The listing builds one solid part. Answer for the finished solid, in the listing's coordinates (mm). Face numbers are marked on the shaded views. Give positions to 0.01 mm unless a question says otherwise; leave off trailing zeros. Loops run counter-clockwise (first coordinate to the right, second up) from the corner with the lowest first, then second, coordinate; pieces in that order, holes last. Notation, with made-up numbers: M 67,74.25 L 81,74.25 A20 ccw 81,86.25 Z; hole C 39.5,-2.5 d4. An arc over 180 degrees is marked long. Return JSON: item names as keys, results as strings.
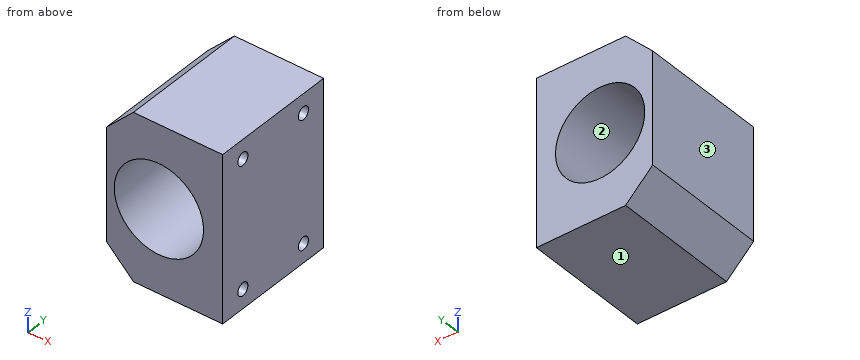
Autodesk Inventor part; units mm, degrees
ref_plane "YZ Plane" through (0, 0, 0) normal (1, 0, 0) x (0, 1, 0)
ref_plane "XZ Plane" through (0, 0, 0) normal (0, 1, 0) x (-1, 0, 0)
ref_plane "XY Plane" through (0, 0, 0) normal (0, 0, 1) x (1, 0, 0)
sketch "Sketch1" plane through (0, 0, 0) normal (0, 1, 0) x (-1, 0, 0)
  circle A0 centre (0, 0) radius 14
  line L0 (0, 0) -> (-20, 0)
  line L1 (-20, 0) -> (-20, -26)
  line L2 (-20, -26) -> (8, -26)
  line L3 (8, -26) -> (16.4853, -17.5147)
  line L4 (-20, 0) -> (-20, 26)
  line L5 (-20, 26) -> (8, 26)
  line L6 (8, 26) -> (16.4853, 17.5147)
  line L7 (16.4853, 17.5147) -> (16.4853, -17.5147)
  dimension "d0" = 28
  dimension "d1" = 20
  dimension "d2" = 26
  dimension "d3" = 28
  dimension "d4" = 12
  dimension "d5" = 135
  dimension "d6" = 28
  dimension "d7" = 26
  dimension "d8" = 12
extrude "Extrusion1" add sketch "Sketch1" along normal blind 40
sketch "Sketch2" plane through (20, 0, 26) normal (1, 0, 0) x (0, 0, -1)
  line L0 (0, 0) -> (0, 40)
  line L1 (0, 40) -> (0, 32)
  circle A0 centre (6, 32) radius 2
  point P0 (26, 0)
  dimension "d11" = 8
  dimension "d13" = 4
extrude "Extrusion2" cut sketch "Sketch2" against normal blind 15
pattern_linear "Rectangular Pattern1" count 2 spacing 24 along (0, -1, 0) count 2 spacing 40 along (0, 0, -1) of "Extrusion2"
properties part number "Soporte Tuerca"
(1) Straight lines are drawn through the part: line 1 along Y through (x, z) = (8.25, 20); line 2 along Y through (x, z) = (7.5, 21.5); line 3 along Z through (x, y) = (0, 11). For each, find the intervals that lie inside material, in ascending order.
Values follow:
{"line 1": "0 to 6, 10 to 30, 34 to 40", "line 2": "0 to 6.68, 9.32 to 30.68, 33.32 to 40", "line 3": "-26 to -14, 14 to 26"}
(2) The part is cut by section A-A (x = 0). Determine the outline of the cut face in (y, z), and give its area (3 significant figures).
Values follow:
{"outline": "M 0,-26 L 40,-26 L 40,-14 L 0,-14 Z; M 0,14 L 40,14 L 40,26 L 0,26 Z", "area": "960 mm²"}
(3) The part is cut by section C-C (z = 0). Determine the outline of the cut face in (x, y).
Values follow:
{"outline": "M -16.49,0 L -14,0 L -14,40 L -16.49,40 Z; M 14,0 L 20,0 L 20,40 L 14,40 Z"}
(4) Determine the mould class of the marked faces 1, 2 and 3 for opening direction Z: released by +Z, released by -Z, zero draft, split by the parting line, or undercut.
Values follow:
{"face 1": "released by -Z", "face 2": "undercut", "face 3": "zero draft"}
(5) The part is cut by section D-D (x = 11). Determine the outline of the cut face in (y, z).
Values follow:
{"outline": "M 0,-26 L 40,-26 L 40,-8.66 L 0,-8.66 Z; M 0,8.66 L 40,8.66 L 40,26 L 0,26 Z; hole C 8,-20 d4; hole C 8,20 d4; hole C 32,-20 d4; hole C 32,20 d4"}
(6) The part is cut by section B-B (y = 19.5). Determine the outline of the cut face in (x, z).
Values follow:
{"outline": "M -16.49,-17.51 L -8,-26 L 20,-26 L 20,26 L -8,26 L -16.49,17.51 Z; hole C 0,0 d28"}
(7) Given pin 1 (3.5 mm diameter, centred on y = 32, z = -20, fed in from -X); pin 2 (1 mm diameter, centred on y = 31, z = -19.5, fed in from +X), each flat-ended and moving along its own axis, determine where each tip first touches the part or whether it passes through.
Values follow:
{"pin 1": "x = -15.75", "pin 2": "x = 5"}
